Source: CAD feature listing. Evaluate the final solid. Frame: model axes, mm. Face numbers are marked on the shaded views. A direction names the side the tool comes from. Coordinates: 2 decimals unless noted, no trailing zeros. Loops run counter-clockwise (first coordinate to the right, second up) from the corner with the lowest first, then second, coordinate; pieces in that order, holes last. Notation, with made-up numbers: (71, 51.25) - (78, 51.25) arc R21 cw to (78, 57.25) - close; hole circle Ø10 at (-3, 26). An arc over 180 degrees is marked (long way). Use one line per item in the form item = value. Start each with the question number.
from build123d import *

# Parameters (mm, degrees)
SKETCH_2_W          = 40
SKETCH_2_H          = 39
EXTRUDE_1_DEPTH     = 20
SKETCH_3_R          = 4
EXTRUDE_2_DEPTH     = 1
SKETCH_4_R          = 3.5
EXTRUDE_3_DEPTH     = 0.5
SKETCH_6_R          = 3
EXTRUDE_4_DEPTH     = 4.5
SKETCH_7_W          = 20
SKETCH_7_H          = 3
EXTRUDE_5_DEPTH     = 6
SKETCH_8_R          = 2
CUT_EXTRUDE_1_DEPTH = 6
FILLET_6_R          = 1
FILLET_7_R          = 1
FILLET_8_R          = 1
FILLET_9_R          = 1
FILLET_10_R         = 1
FILLET_11_R         = 1
FILLET_12_R         = 1


with BuildPart() as part:
    # 草图2 → 凸台-拉伸1 (new body)
    with BuildSketch(Plane.XY):
        Rectangle(SKETCH_2_W, SKETCH_2_H)
    extrude(amount=EXTRUDE_1_DEPTH)

    # 草图3 → 凸台-拉伸2 (add)
    with BuildSketch(Plane(origin=(0, 19.5, 0), x_dir=(1, 0, 0), z_dir=(0, 1, 0))):
        with Locations(Location((-9, -10, 0), (0, 0, 90))):
            Circle(SKETCH_3_R)
    extrude(amount=EXTRUDE_2_DEPTH)

    # 草图4 → 凸台-拉伸3 (add)
    with BuildSketch(Plane(origin=(0, 20.5, 0), x_dir=(1, 0, 0), z_dir=(0, 1, 0))):
        with Locations(Location((-9, -10, 0), (0, 0, 270))):
            Circle(SKETCH_4_R)
    extrude(amount=EXTRUDE_3_DEPTH)

    # 草图6 → 凸台-拉伸4 (add)
    with BuildSketch(Plane(origin=(0, 21, 0), x_dir=(1, 0, 0), z_dir=(0, 1, 0))):
        with Locations(Location((-9, -10, 0), (0, 0, 270))):
            Circle(SKETCH_6_R)
    extrude(amount=EXTRUDE_4_DEPTH)

    # 草图7 → 凸台-拉伸5 (add)
    with BuildSketch(Plane.ZY.offset(20)):
        with Locations((10, 10)):
            Rectangle(SKETCH_7_W, SKETCH_7_H)
    extrude_5 = extrude(amount=EXTRUDE_5_DEPTH)

    # 草图8 → 切除-拉伸1 (cut)
    with BuildSketch(Plane(origin=(0, 11.5, 0), x_dir=(1, 0, 0), z_dir=(0, 1, 0))):
        with Locations(Location((-23, -4.880823414, 0), (0, 0, 180))):
            Circle(SKETCH_8_R)
        with Locations(Location((-23, -14.880823414, 0), (0, 0, 180))):
            Circle(SKETCH_8_R)
    cut_extrude_1 = extrude(amount=-CUT_EXTRUDE_1_DEPTH, mode=Mode.SUBTRACT)

    # 镜向3: 凸台-拉伸5, 切除-拉伸1 across plane
    add(extrude_5.mirror(Plane(origin=(0, 0, 0), x_dir=(0, 0, 1), z_dir=(1, 0, 0))))
    add(cut_extrude_1.mirror(Plane(origin=(0, 0, 0), x_dir=(0, 0, 1), z_dir=(1, 0, 0))), mode=Mode.SUBTRACT)

    # 圆角6
    fillet_6_edges = [part.edges().sort_by_distance(p)[0] for p in [
        (-20, -19.5, 10),
    ]]
    fillet(fillet_6_edges, radius=FILLET_6_R)

    # 圆角7
    fillet_7_edges = [part.edges().sort_by_distance(p)[0] for p in [
        (20, -19.5, 10),
    ]]
    fillet(fillet_7_edges, radius=FILLET_7_R)

    # 圆角8
    fillet_8_edges = [part.edges().sort_by_distance(p)[0] for p in [
        (20, 19.5, 10),
    ]]
    fillet(fillet_8_edges, radius=FILLET_8_R)

    # 圆角9
    fillet_9_edges = [part.edges().sort_by_distance(p)[0] for p in [
        (-20, 19.5, 10),
    ]]
    fillet(fillet_9_edges, radius=FILLET_9_R)

    # 圆角10
    fillet_10_edges = [part.edges().sort_by_distance(p)[0] for p in [
        (-26, 10, 20),
        (-26, 10, 0),
    ]]
    fillet(fillet_10_edges, radius=FILLET_10_R)

    # 圆角11
    fillet_11_edges = [part.edges().sort_by_distance(p)[0] for p in [
        (26, 10, 0),
        (26, 10, 20),
    ]]
    fillet(fillet_11_edges, radius=FILLET_11_R)

    # 圆角12
    fillet_12_edges = [part.edges().sort_by_distance(p)[0] for p in [
        (-20, 15, 20),
        (-20, 15, 0),
        (-19.707106781, 19.207106781, 0),
        (-19.707106781, 19.207106781, 20),
        (-20, -5, 0),
        (-20, -5, 20),
        (20, 15, 0),
        (20, 15, 20),
        (0, -19.5, 0),
        (0, -19.5, 20),
        (-19.707106781, -19.207106781, 0),
        (-19.707106781, -19.207106781, 20),
        (20, -5, 20),
        (20, -5, 0),
        (19.707106781, -19.207106781, 0),
        (19.707106781, -19.207106781, 20),
        (0, 19.5, 0),
        (0, 19.5, 20),
        (19.707106781, 19.207106781, 0),
        (19.707106781, 19.207106781, 20),
    ]]
    fillet(fillet_12_edges, radius=FILLET_12_R)


solid = part.part
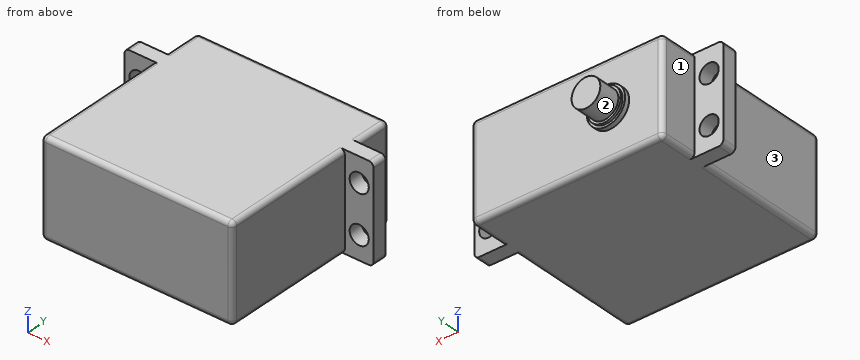
(1) Cut plane B-B, the plane y = -2.5. Output: boundary loops of the cut face in (x, z).
(2) Access query for the marked faces 1, 2 and 3. Directions: +Z, -Z, +X, -X, +Y, -Y. A direction counts if a zero-diameter tool reaches every point of the face in a straight line with its end or side. Return the directions, or none.
(3) Cut plane C-C, the plane x = -17. Output: boundary loops of the cut face in (y, z), plus the area to 3 significant figures.
(4) Material intervals for line 1 (Z direction, x = -23, y = 10.8); line 2 (Y direction, x = -14, z = 17.75); line 3 (X direction, y = 2, z = 4.75), sorted ascending.
(5) Contact query for flat-ended pins moving along their axis: pin 1 (6.5 mm diameter, centred on x = -23, z = 14.88, fed in from +Y); pin 2 (7.5 mm diameter, centred on x = -24, z = 6.5, fed in from -Y); pin 3 (1.5 mm diameter, centred on y = 4, z = 16, fed in from +X); pin 4 (3 mm diameter, centred on x = -23, z = 4.88, fed in from +Y). Output: stop coordinate, or through.
(6) Cut plane D-D, the plane z = 10. Output: boundary loops of the cut face in (x, y), plus the area to 3 significant figures.
(7) Cut plane A-A, the plane x = 23. Output: boundary loops of the cut face in (y, z), plus the area to 3 significant figures.
Recorded:
q1.outline = (-20, 1) arc R1 ccw to (-19, 0) - (19, 0) arc R1 ccw to (20, 1) - (20, 19) arc R1 ccw to (19, 20) - (-19, 20) arc R1 ccw to (-20, 19) - close
q2.face_1 = +Z, -Z, -X, +Y
q2.face_2 = +Y
q2.face_3 = +Z, -Z, -X, -Y
q3.outline = (-19.5, 1) arc R1 ccw to (-18.5, 0) - (18.5, 0) arc R1 ccw to (19.5, 1) - (19.5, 19) arc R1 ccw to (18.5, 20) - (-18.5, 20) arc R1 ccw to (-19.5, 19) - close
q3.area = 779 mm²
q4.line_1 = 0 to 2.88, 6.88 to 12.88, 16.88 to 20
q4.line_2 = -19.5 to 19.5
q4.line_3 = -20 to 20
q5.pin_1 = 19.16
q5.pin_2 = 8.5
q5.pin_3 = 20
q5.pin_4 = through
q6.outline = (-26, 8.5) - (-20, 8.5) - (-20, -18.5) arc R1 ccw to (-19, -19.5) - (19, -19.5) arc R1 ccw to (20, -18.5) - (20, 8.5) - (26, 8.5) - (26, 11.5) - (20, 11.5) - (20, 18.5) arc R1 ccw to (19, 19.5) - (-5, 19.5) - (-5, 20.5) - (-5.5, 20.5) - (-5.5, 21) - (-6, 21) - (-6, 25.5) - (-12, 25.5) - (-12, 21) - (-12.5, 21) - (-12.5, 20.5) - (-13, 20.5) - (-13, 19.5) - (-19, 19.5) arc R1 ccw to (-20, 18.5) - (-20, 11.5) - (-26, 11.5) - close
q6.area = 1,630 mm²
q7.outline = (8.5, 0) - (11.5, 0) - (11.5, 2.88) - (8.5, 2.88) - close; (8.5, 6.88) - (11.5, 6.88) - (11.5, 12.88) - (8.5, 12.88) - close; (8.5, 16.88) - (11.5, 16.88) - (11.5, 20) - (8.5, 20) - close
q7.area = 36.0 mm²
